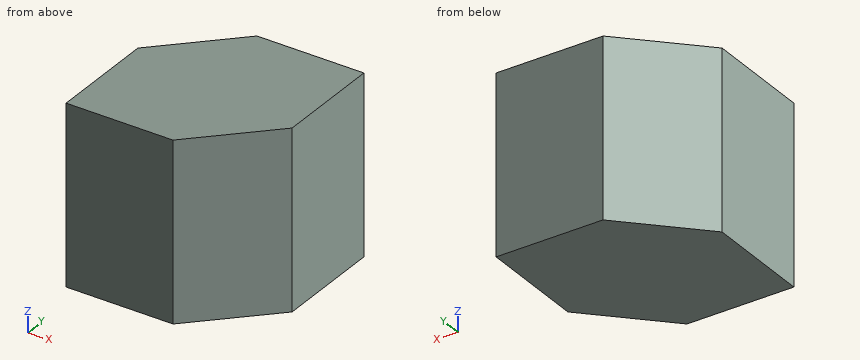
from build123d import *

# Parameters (mm, degrees)
F0_W     = 127
F0_H     = 127
F1_DEPTH = 101.6
F3_DEPTH = 101.6
F4_DEPTH = 25.4


with BuildPart() as f1:
    # F0 (on Top) → F1 (new body)
    with BuildSketch(Plane.XY):
        Rectangle(F0_W, F0_H)
    extrude(amount=F1_DEPTH)

    # F2 (on face) → F3 (cut)
    with BuildSketch(Plane.XY.offset(101.6)):
        Polygon((-12.7, 63.5), (-63.5, 63.5), (-63.5, 12.7), align=None)
        Polygon((63.5, -63.5), (63.5, -12.7), (12.7, -63.5), align=None)
    extrude(amount=-F3_DEPTH, mode=Mode.SUBTRACT)

    # F1_face (on face) → F4 (join)
    with BuildSketch(Plane.XY.offset(101.6)):
        Polygon((63.5, -12.7), (63.5, 63.5), (-12.7, 63.5), (-63.5, 12.7), (-63.5, -63.5), (12.7, -63.5), align=None)
    extrude(amount=F4_DEPTH)


solid = f1.part
Read the model definition and answer for the solid it produces. Units are mm, in the model's axes. Round coordinates to 2 decimals unless told otherwise and drop trailing zeros. Write each loop counter-clockwise with the first axis right and the second up, starting at its lowest first coordinate (ties: lowest second). Pieces come first, ordered by that corner, then holes.
1. The part is cut by section B-B, the plane z = 22. Determine the outline of the cut face in (x, y).
2. The part is cut by section A-A, the plane x = -33.5. Determine the outline of the cut face in (y, z).
3. Given pin 1 Ø10 at (y, z) = (-35.5, 100) entering from +X, flat-ended and moving along its own axis, determine where the tip first touches the part or whether it passes through.
4. The part is cut by section C-C, the plane y = -32.5. Determine the outline of the cut face in (x, z), then the cut area to 3 significant figures.
5. Straight lines are drawn through the part: L1, parallel to X at y = 53, z = 73; L2, parallel to Y at x = 21.5, z = 11; L3, parallel to Y at x = 20, z = 40. For each, find the intervals that lie inside material, in ascending order.
Values:
1. outline: (-63.5, -63.5) - (12.7, -63.5) - (63.5, -12.7) - (63.5, 63.5) - (-12.7, 63.5) - (-63.5, 12.7) - close
2. outline: (-63.5, 0) - (42.7, 0) - (42.7, 127) - (-63.5, 127) - close
3. pin 1: stops at x = 45.7
4. outline: (-63.5, 0) - (43.7, 0) - (43.7, 127) - (-63.5, 127) - close
4. area: 13,600 mm2
5. L1: x = -23.2 to 63.5
5. L2: y = -54.7 to 63.5
5. L3: y = -56.2 to 63.5
